Part print with two shaded views. Sizes in mm from the minimum x, y, z corner. A direction names the side the tool comes from. Round coordinates to 2 decimals unless told otherwise and drop trailing zeros. Write each loop counter-clockwise with the first axis right and the second up, starting at its lowest first coordinate (ties: lowest second). Pieces come first, ordered by that corner, then holes. Notation, with made-up numbers: M 4,3.25 L 43,3.25 A15 cw 43,30.25 Z; hole C -6,84.5 d1. An arc over 180 degrees is marked long. Use one line per item in the form item = value. Start each with the question number.
Item 1: Probe L1, parallel to Y at x = 4, z = 1.5; L2, parallel to X at y = 44, z = 1.3; L3, parallel to Y at x = 25, z = 1. List the from-to ranges inside material, lowest first.
Item 2: Flat gauge pins, fed straight in: pin 1 Ø2 at (x, y) = (24, 44) entering from +Z; pin 2 Ø3 at (x, z) = (24.5, 5.5) entering from +Y; pin 3 Ø1 at (x, z) = (14.5, 3.5) entering from -Y; pin 4 Ø4 at (x, y) = (4, 4) entering from +Z. Where does each tip first touch, or does it go through?
Item 3: Cut at D-D, the plane y = 31. Give the cut face in (x, z).
Item 4: Cut at A-A, the plane y = 4. Give the cut face in (x, z).
Item 5: Cut at C-C, the plane x = 19.5. Give the cut face in (y, z), then the cut area to 3 significant figures.
Item 6: Cut at B-B, the plane x = 4. Give the cut face in (y, z), then the cut area to 3 significant figures.
Item 7: Which spindle directions (+Z, -Z, +X, -X, +Y, -Y) get a long thin tool onto all of the face, cutting with end or side? Do the marked faces 1, 2 and 3. Say none if no direction does.
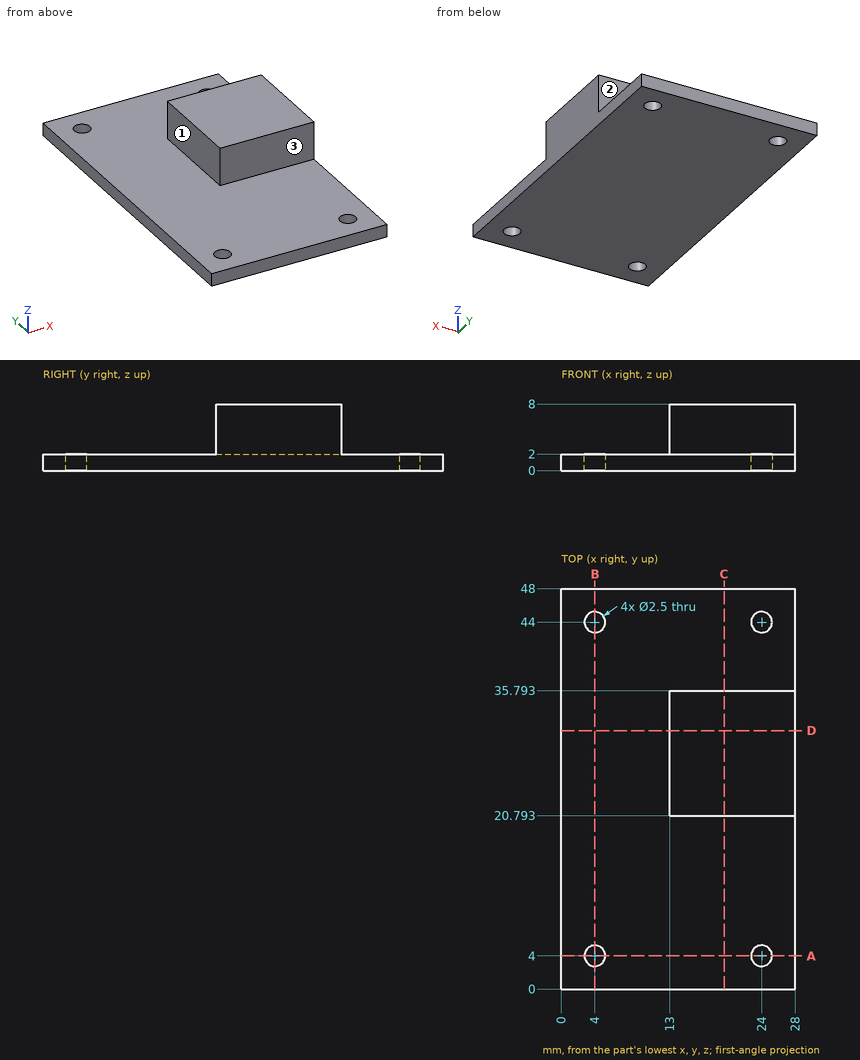
Model answer:
q1.L1 = 0 to 2.75, 5.25 to 42.75, 45.25 to 48
q1.L2 = 0 to 2.75, 5.25 to 22.75, 25.25 to 28
q1.L3 = 0 to 3.25, 4.75 to 43.25, 44.75 to 48
q2.pin_1 = through
q2.pin_2 = 35.79
q2.pin_3 = 20.79
q2.pin_4 = 2
q3.outline = M 0,0 L 28,0 L 28,8 L 13,8 L 13,2 L 0,2 Z
q4.outline = M 0,0 L 2.75,0 L 2.75,2 L 0,2 Z; M 5.25,0 L 22.75,0 L 22.75,2 L 5.25,2 Z; M 25.25,0 L 28,0 L 28,2 L 25.25,2 Z
q5.outline = M 0,0 L 48,0 L 48,2 L 35.79,2 L 35.79,8 L 20.79,8 L 20.79,2 L 0,2 Z
q5.area = 186 mm²
q6.outline = M 0,0 L 2.75,0 L 2.75,2 L 0,2 Z; M 5.25,0 L 42.75,0 L 42.75,2 L 5.25,2 Z; M 45.25,0 L 48,0 L 48,2 L 45.25,2 Z
q6.area = 86.0 mm²
q7.face_1 = +Z, -X, +Y, -Y
q7.face_2 = +Z, +X, -X, +Y
q7.face_3 = +Z, +X, -X, -Y
